from build123d import *

# Parameters (mm, degrees)
SKETCH1_R           = 2.5527
BOSS_EXTRUDE1_DEPTH = 6.35


with BuildPart() as part:
    # Sketch1 → Boss-Extrude1 (new body)
    with BuildSketch(Plane.XY):
        with BuildLine():
            Line((-17.751257214, 44.45), (-20.0152, 44.45))
            ThreePointArc((-20.0152, 44.45), (-22.709276836, 43.334076836), (-23.8252, 40.64))
            Line((-23.8252, 40.64), (-23.8252, 10.16))
            ThreePointArc((-23.8252, 10.16), (-22.709276836, 7.465923164), (-20.0152, 6.35))
            Line((-20.0152, 6.35), (-8.200857214, 6.35))
            ThreePointArc((-8.200857214, 6.35), (-5.134034416, 4.800685279), (-4.561423539, 1.412781065))
            ThreePointArc((-4.561423539, 1.412781065), (0, -4.7752), (4.561423539, 1.412781065))
            ThreePointArc((4.561423539, 1.412781065), (5.134034416, 4.800685279), (8.200857214, 6.35))
            Line((8.200857214, 6.35), (10.4648, 6.35))
            ThreePointArc((10.4648, 6.35), (13.158876836, 7.465923164), (14.2748, 10.16))
            Line((14.2748, 10.16), (14.2748, 19.05))
            Line((14.2748, 19.05), (9.398, 19.05))
            ThreePointArc((9.398, 19.05), (8.320369265, 19.496369265), (7.874, 20.574))
            Line((7.874, 20.574), (7.874, 30.226))
            ThreePointArc((7.874, 30.226), (8.320369265, 31.303630735), (9.398, 31.75))
            Line((9.398, 31.75), (14.2748, 31.75))
            Line((14.2748, 31.75), (14.2748, 40.64))
            ThreePointArc((14.2748, 40.64), (13.158876836, 43.334076836), (10.4648, 44.45))
            Line((10.4648, 44.45), (-1.349542786, 44.45))
            ThreePointArc((-1.349542786, 44.45), (-4.416365584, 45.999314721), (-4.988976461, 49.387218935))
            ThreePointArc((-4.988976461, 49.387218935), (-9.5504, 55.5752), (-14.111823539, 49.387218935))
            ThreePointArc((-14.111823539, 49.387218935), (-14.684434416, 45.999314721), (-17.751257214, 44.45))
        make_face()
        Circle(SKETCH1_R, mode=Mode.SUBTRACT)
        with Locations((-9.5504, 50.8)):
            Circle(SKETCH1_R, mode=Mode.SUBTRACT)
        with BuildLine():
            ThreePointArc((-7.9248, 30.226), (-7.478430735, 31.303630735), (-6.4008, 31.75))
            Line((-6.4008, 31.75), (-1.524, 31.75))
            ThreePointArc((-1.524, 31.75), (-0.446369265, 31.303630735), (0, 30.226))
            Line((0, 30.226), (0, 20.574))
            ThreePointArc((0, 20.574), (-0.446369265, 19.496369265), (-1.524, 19.05))
            Line((-1.524, 19.05), (-6.4008, 19.05))
            ThreePointArc((-6.4008, 19.05), (-7.478430735, 19.496369265), (-7.9248, 20.574))
            Line((-7.9248, 20.574), (-7.9248, 30.226))
        make_face(mode=Mode.SUBTRACT)
    extrude(amount=BOSS_EXTRUDE1_DEPTH)


solid = part.part
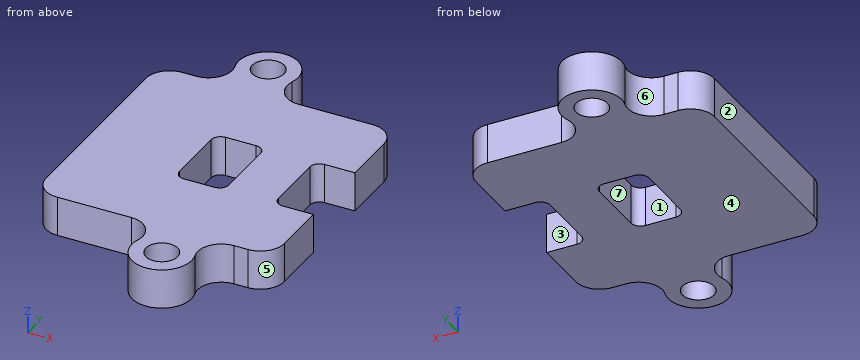
Read the model definition and answer for the solid it produces. Units are mm, in the model's axes. Face numbers are marked on the shaded views. A direction names the side the tool comes from. Give positions to 0.01 mm unless a question says otherwise; leave off trailing zeros. Write each loop counter-clockwise with the first axis right and the second up, starting at its lowest first coordinate (ties: lowest second). Pieces come first, ordered by that corner, then holes. Notation, with made-up numbers: (24.25, 30) - (40.25, 30) arc R20 ccw to (40.25, 39) - close; hole circle Ø1 at (3, 24). An arc over 180 degrees is marked (long way). Answer in a Markdown table with one row per item. Add a question column.
Item 1: A tool of negligible diameter and unlimited length cuts with its end or side. For the marked faces 1, 2 and 3, from which of +Z, -Z, +X, -X, +Y, -Y can it reach the whole face along a straight path? Write none if from no direction.
Item 2: Determine the mould class of the marked faces 4, 5, 6 and 7 for opening direction Y: pulls with the +Y half, pulls with the -Y half, needs draft (parallel to the pull), parting line crosses it, or undercut.
Item 3: Find the intervals of material crossed by L1, parallel to Y at x = -9.5, z = 1.75; L2, parallel to X at y = 29, z = 4.5; L3, parallel to X at y = 48.5, z = 0.75, in increasing order.
Item 4: Section A-A, the plane y = 50.8 is taken. Write down the section's boundary in (x, z).
Item 5: Flat-ended cylindrical pins translate along their axes: P1, Ø1.1, axis at x = 9, z = 3.5, coming from the -Y side; P2, Ø1.1, axis at x = -19, z = 4, coming from the +Y side; P3, Ø1.5, axis at x = -5, z = 3.5, coming from the -Y side. Find the tip coordinate at first contact, or state that the pin passes through.
Item 6: Section B-B, the plane z = 3.25 is taken. Count the separate pieces of the cut face and the enclosed holes in it, and give its area (3 significant figures).
Recorded:
| question | item | result |
|---|---|---|
| 1 | face 1 | +Z, -Z |
| 1 | face 2 | +Z, -Z, -X, +Y, -Y |
| 1 | face 3 | +Z, -Z, +X |
| 2 | face 4 | needs draft |
| 2 | face 5 | pulls with the -Y half |
| 2 | face 6 | undercut |
| 2 | face 7 | undercut |
| 3 | L1 | y = 6.35 to 48.25, 53.35 to 55.57 |
| 3 | L2 | x = -23.83 to -7.92, 0 to 7.87 |
| 3 | L3 | x = -13.95 to -10.66, -8.44 to -5.15 |
| 4 | outline | (-14.33, 0) - (-12.1, 0) - (-12.1, 6.35) - (-14.33, 6.35) - close; (-7, 0) - (-4.78, 0) - (-4.78, 6.35) - (-7, 6.35) - close |
| 5 | P1 | stops at y = 6.35 |
| 5 | P2 | stops at y = 44.45 |
| 5 | P3 | stops at y = -2.18 |
| 6 | separate pieces | 1 |
| 6 | enclosed holes | 3 |
| 6 | area | 1,420 mm2 |
